Drawing for the job (mm, zero at the part's lowest x, y, z). Give positions to 0.01 mm unless a question says otherwise; leave off trailing zeros. Loops run counter-clockwise (first coordinate to the right, second up) from the corner with the lowest first, then second, coordinate; pieces in that order, holes last. Notation, with made-up numbers: (-7, -9.75) - (6, -9.75) arc R8 cw to (6, -3.75) - close; hole circle Ø1 at (11.5, 61). An arc over 180 degrees is marked (long way). Return JSON: item names as keys, results as strings. Group by question number.
1) Drill centre lines: probe 1 along X at (y, z) = (5, 209.55); probe 2 along X at (y, z) = (5.25, 202); probe 3 along X at (y, z) = (0.5, 125). Where is each one in solid material? Low to high. Write a range as from..to.
2) Slice it at B-B (z = 209.55). List the corners of the cut face in (x, y).
3) Slice it at A-A (z = 136). List the corners of the cut face in (x, y), and give its area (3 significant figures).
4) Slice it at C-C (y = 1.5). Count the separate pieces of the cut face and the enclosed holes in it, and give its area (3 significant figures).
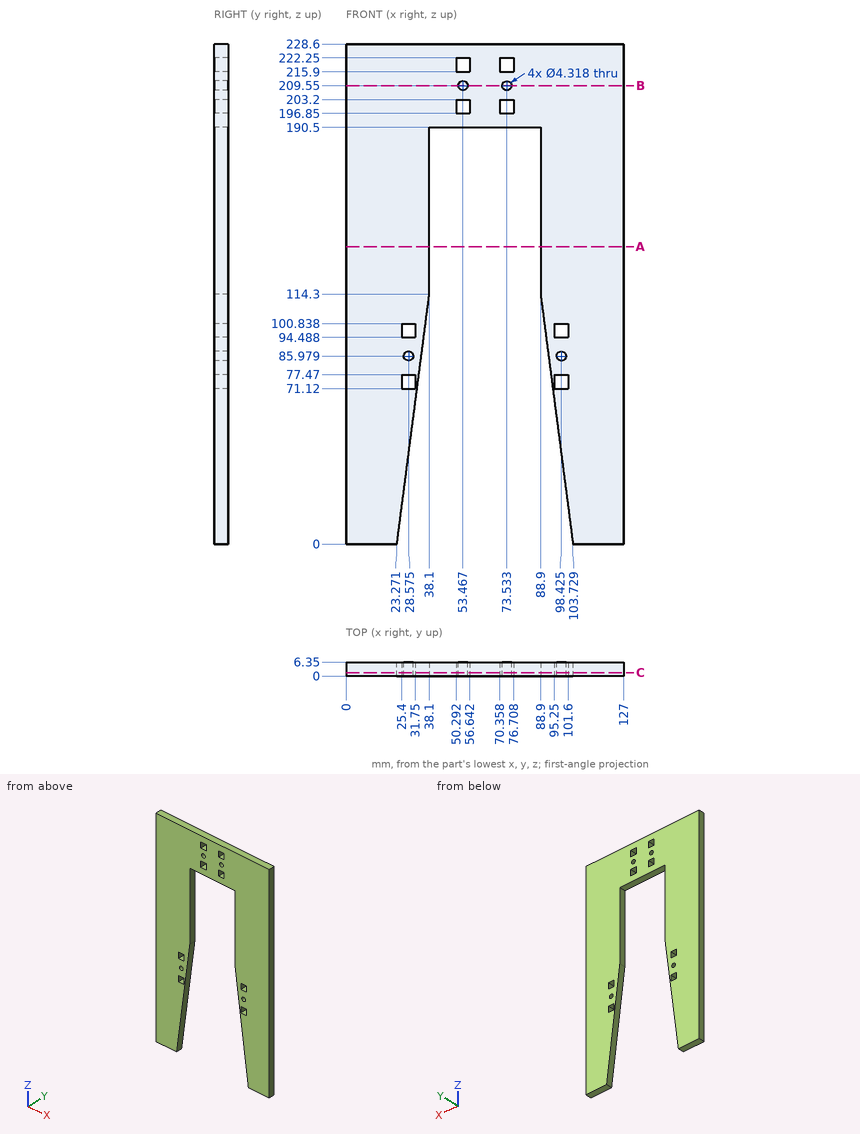
Results:
{
 "1": {"probe 1": "0..51.31, 55.63..71.37, 75.69..127", "probe 2": "0..50.29, 56.64..70.36, 76.71..127", "probe 3": "0..38.1, 88.9..127"},
 "2": {"outline": "(0, 0) - (51.31, 0) - (51.31, 6.35) - (0, 6.35) - close; (55.63, 0) - (71.37, 0) - (71.37, 6.35) - (55.63, 6.35) - close; (75.69, 0) - (127, 0) - (127, 6.35) - (75.69, 6.35) - close"},
 "3": {"outline": "(0, 0) - (38.1, 0) - (38.1, 6.35) - (0, 6.35) - close; (88.9, 0) - (127, 0) - (127, 6.35) - (88.9, 6.35) - close", "area": "484 mm2"},
 "4": {"separate pieces": "1", "enclosed holes": "12", "area": "17,300 mm2"}
}
